from build123d import *

# Parameters (mm, degrees)
CROQUIS1_R              = 13
SALIENTE_EXTRUIR1_DEPTH = 1
CROQUIS2_R              = 3.95
SALIENTE_EXTRUIR2_DEPTH = 3.5
CROQUIS3_R              = 2.6
CORTAR_EXTRUIR1_DEPTH   = 19.927493231


with BuildPart() as part:
    # Croquis1 → Saliente-Extruir1 (new body)
    with BuildSketch(Plane(origin=(0, 0, 0), x_dir=(1, 0, 0), z_dir=(0, 1, 0))):
        with Locations(Location((0, 0, 0), (0, 0, 270))):
            Circle(CROQUIS1_R)
    extrude(amount=SALIENTE_EXTRUIR1_DEPTH)

    # Croquis2 → Saliente-Extruir2 (add)
    with BuildSketch(Plane(origin=(0, 1, 0), x_dir=(1, 0, 0), z_dir=(0, 1, 0))):
        with Locations(Location((0, 0, 0), (0, 0, 270))):
            Circle(CROQUIS2_R)
    extrude(amount=SALIENTE_EXTRUIR2_DEPTH)

    # Croquis3 → Cortar-Extruir1 (cut, through all)
    with BuildSketch(Plane(origin=(0, 4.5, 0), x_dir=(1, 0, 0), z_dir=(0, 1, 0))):
        with Locations(Location((0, 0, 0), (0, 0, 270))):
            Circle(CROQUIS3_R)
    extrude(amount=-CORTAR_EXTRUIR1_DEPTH, mode=Mode.SUBTRACT)


solid = part.part
The model under review builds one solid part; all positions refer to its coordinate system, in mm. Round coordinates to 2 decimals unless told otherwise and drop trailing zeros. Write each loop counter-clockwise with the first axis right and the second up, starting at its lowest first coordinate (ties: lowest second). Pieces come first, ordered by that corner, then holes. Notation, with made-up numbers: M -9.75,67.25 L 9.25,67.25 A21 ccw 9.25,106.25 Z; hole C 52.25,70.5 d11. An arc over 180 degrees is marked long. Answer as CSV lines item,"result". Start each with the question number.
Q1. Consider section B-B, the plane z = 0. Give the boundary of the cut face in (x, y), then the cut area to 4 significant figures.
Q2. Consider section D-D, the plane z = 3.25. Give the boundary of the cut face in (x, y) (3 decimals).
Q3. Wall thickness on line 1 along X through (y, z) = (3.2, 0); line 2 along Y through (x, z) = (8.75, -5.5); line 3 along X through (y, z) = (0.9, 0): over which ranges is each line inside the solid? List them lowest first.
Q4. Consider section A-A, the plane x = 0. Give the boundary of the cut face in (y, z).
Q5. Clearance check with flat-ended pins moving along their axes: P1, Ø3, axis at x = -5, z = 7.5, coming from the +Y side; P2, Ø1, axis at y = 1, z = -3, coming from the -X side. State where each tip first meets the part, or that it passes through.
Q6. Consider section C-C, the plane y = 0.55. Give the boundary of the cut face in (x, z).
Q7. The part is to be moulded in two halves that separate along Z. For faces 1 (the face through (2.67, 2.73, -2.91)), 2 (the face through (0.78, 2.28, 2.48)), 3 (the face through (3, 1, 3)), say which applies: +Z half, -Z half, draft (parallel to the pull), parting line (faces both ways), or undercut.
Result set:
1,outline,"M -13,0 L -2.6,0 L -2.6,4.5 L -3.95,4.5 L -3.95,1 L -13,1 Z; M 2.6,0 L 13,0 L 13,1 L 3.95,1 L 3.95,4.5 L 2.6,4.5 Z"
1,area,"30.25 mm²"
2,outline,"M -12.587,0 L 12.587,0 L 12.587,1 L 2.245,1 L 2.245,4.5 L -2.245,4.5 L -2.245,1 L -12.587,1 Z"
3,line 1,"x = -3.95 to -2.6, 2.6 to 3.95"
3,line 2,"y = 0 to 1"
3,line 3,"x = -13 to -2.6, 2.6 to 13"
4,outline,"M 0,-13 L 1,-13 L 1,-3.95 L 4.5,-3.95 L 4.5,-2.6 L 0,-2.6 Z; M 0,2.6 L 4.5,2.6 L 4.5,3.95 L 1,3.95 L 1,13 L 0,13 Z"
5,P1,"stops at y = 1"
5,P2,"stops at x = -12.76"
6,outline,"C 0,0 d26; hole C 0,0 d5.2"
7,face 1,"parting line"
7,face 2,"undercut"
7,face 3,"draft"
